Geometry check sheet. Reference: the model listing, model coordinates, mm. Face numbers are marked on the shaded views. A direction names the side the tool comes from. Give positions to 0.01 mm unless a question says otherwise; leave off trailing zeros. Loops run counter-clockwise (first coordinate to the right, second up) from the corner with the lowest first, then second, coordinate; pieces in that order, holes last. Notation, with made-up numbers: (-39.75, 67) - (-3.75, 67) arc R25 cw to (-3.75, 88) - close; hole circle Ø4 at (55, 44). An arc over 180 degrees is marked (long way). One line per question, with ' | ' between items. Start each with the question number.
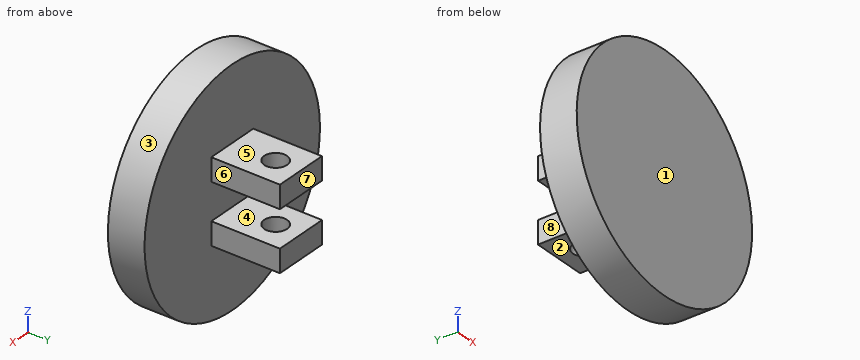
from build123d import *

# Parameters (mm, degrees)
SKETCH1_R           = 250
BOSS_EXTRUDE1_DEPTH = 80
SKETCH2_W           = 120
SKETCH2_H           = 50
SKETCH2_W_2         = 119.52714404
BOSS_EXTRUDE2_DEPTH = 150
SKETCH3_R           = 25
CUT_EXTRUDE1_DEPTH  = 481.624593628


with BuildPart() as part:
    # Sketch1 → Boss-Extrude1 (new body)
    with BuildSketch(Plane(origin=(0, 0, 0), x_dir=(1, 0, 0), z_dir=(0, 1, 0))):
        with Locations(Location((0, 0, 0), (0, 0, 270))):
            Circle(SKETCH1_R)
    extrude(amount=BOSS_EXTRUDE1_DEPTH)

    # Sketch2 → Boss-Extrude2 (add)
    with BuildSketch(Plane(origin=(0, 80, 0), x_dir=(1, 0, 0), z_dir=(0, 1, 0))):
        with Locations((-0.23642798, 65)):
            Rectangle(SKETCH2_W, SKETCH2_H)
        with Locations((0, -65)):
            Rectangle(SKETCH2_W_2, SKETCH2_H)
    extrude(amount=BOSS_EXTRUDE2_DEPTH)

    # Sketch3 → Cut-Extrude1 (cut, through all)
    with BuildSketch(Plane.XY.offset(90)):
        with Locations((0.23642798, 175)):
            Circle(SKETCH3_R)
    extrude(amount=-CUT_EXTRUDE1_DEPTH, mode=Mode.SUBTRACT)


solid = part.part
(1) Section check B-B, the plane y = 175. Record the boundary of the cut face in (x, z), and give its area (3 significant figures).
(2) Section check D-D, the plane z = 0. Record the boundary of the cut face in (x, y), and give its area (3 significant figures).
(3) Mould release check, pull along Z, two halves, no side actions. Record for the marked faces 1, 2, 3 and 4: pulls with the +Z half, pulls with the -Z half, needs draft (parallel to the pull), parting line crosses it, or undercut.
(4) Section check C-C, the plane x = 0. Record the boundary of the cut face in (y, z), and give its area (3 significant figures).
(5) Depth check by flat-ended pin: pin 1 Ø8 at (y, z) = (62.5, -137.5) entering from +X; pin 2 Ø15 at (y, z) = (143, 57) entering from -X; pin 3 Ø2 at (x, y) = (37, 42.5) entering from -Z. Enter the tip coordinate at first touch or a pass-through.
(6) Tool access check on the marked faces 5, 6, 7 and 8. Record the directions out of +Z, -Z, +X, -X, +Y, -Y that give a thin tool (end or side, any length) a straight path to the whole face; none if there is none.
(7) Section check A-A, the plane y = 100. Record the boundary of the cut face in (x, z).
(8) Material ranges on line 1 (Z direction, x = -9.5, y = 142); line 2 (Y direction, x = 8, z = 141); line 3 (X direction, y = 122, z = 65), recorded low to high.
Numbers:
1) outline: (-60.24, -90) - (-24.76, -90) - (-24.76, -40) - (-60.24, -40) - close; (-59.76, 40) - (-24.76, 40) - (-24.76, 90) - (-59.76, 90) - close; (25.24, -90) - (59.76, -90) - (59.76, -40) - (25.24, -40) - close; (25.24, 40) - (59.76, 40) - (59.76, 90) - (25.24, 90) - close | area: 6,980 mm^2
2) outline: (-250, 0) - (250, 0) - (250, 80) - (-250, 80) - close | area: 40,000 mm^2
3) face 1: needs draft | face 2: pulls with the -Z half | face 3: parting line crosses it | face 4: undercut
4) outline: (0, -250) - (80, -250) - (80, -90) - (150, -90) - (150, -40) - (80, -40) - (80, 40) - (150, 40) - (150, 90) - (80, 90) - (80, 250) - (0, 250) - close; (200, -90) - (230, -90) - (230, -40) - (200, -40) - close; (200, 40) - (230, 40) - (230, 90) - (200, 90) - close | area: 50,000 mm^2
5) pin 1: x = 211.37 | pin 2: x = -59.76 | pin 3: z = -247.39
6) face 5: +Z, +X, -X, +Y | face 6: +Z, -Z, +X, +Y | face 7: +Z, -Z, +X, -X, +Y | face 8: +Z, -Z, -X, +Y
7) outline: (-60.24, -90) - (59.76, -90) - (59.76, -40) - (-60.24, -40) - close; (-59.76, 40) - (59.76, 40) - (59.76, 90) - (-59.76, 90) - close
8) line 1: -90 to -40, 40 to 90 | line 2: 0 to 80 | line 3: -59.76 to 59.76
